from build123d import *

# Parameters (mm, degrees)
SALIENTE_EXTRUIR1_DEPTH = 3
CROQUIS2_R              = 2.5
CROQUIS2_R_2            = 1.1
CORTAR_EXTRUIR1_DEPTH   = 10
REDONDEO1_R             = 5


with BuildPart() as part:
    # Croquis1 → Saliente-Extruir1 (new body)
    with BuildSketch(Plane(origin=(0, 0, 0), x_dir=(1, 0, 0), z_dir=(0, 1, 0))):
        Polygon((-6, 5), (-6, 2.5), (-9, 2.5), (-9, -2.5), (-6, -2.5), (-6, -5), (6, -5), (6, 5), align=None)
    extrude(amount=SALIENTE_EXTRUIR1_DEPTH)

    # Croquis2 → Cortar-Extruir1 (cut)
    with BuildSketch(Plane(origin=(0, 3, 0), x_dir=(1, 0, 0), z_dir=(0, 1, 0))):
        with Locations(Location((1.4, 0, 0), (0, 0, 270))):
            Circle(CROQUIS2_R)
        with Locations(Location((-3.6, 0, 0), (0, 0, 270))):
            Circle(CROQUIS2_R_2)
    extrude(amount=-CORTAR_EXTRUIR1_DEPTH, mode=Mode.SUBTRACT)

    # Redondeo1
    redondeo1_edges = [part.edges().sort_by_distance(p)[0] for p in [
        (6, 1.5, -5),
        (6, 1.5, 5),
    ]]
    fillet(redondeo1_edges, radius=REDONDEO1_R - 0.0001)  # a hair under: the kernel refuses the full size


solid = part.part
Source: CAD feature listing. Evaluate the final solid. Frame: model axes, mm. A direction names the side the tool comes from. Round coordinates to 2 decimals unless told otherwise and drop trailing zeros. Loops run counter-clockwise (first coordinate to the right, second up) from the corner with the lowest first, then second, coordinate; pieces in that order, holes last. Notation, with made-up numbers: (85.5, 83) - (109.5, 83) arc R27 cw to (109.5, 111) - close; hole circle Ø11 at (-15.5, 84.5). An arc over 180 degrees is marked (long way). Write item = value, one per line. Start each with the question number.
Item 1: Reachability of faces 4 (the face through (-8, 1, 2.5)), 5 (the face through (-2.51, 1.52, -0.14)), 6 (the face through (-7, 1, -2.5)) from +Z, -Z, +X, -X, +Y, -Y: full face, straight path, thin tool, end or side. Return the list, or none.
Item 2: Section query B-B on y = 2.35. Count the separate pieces of the cut face and the enclosed holes in it, plus the area to 3 significant figures.
Item 3: Material intervals for line 1 (X direction, y = 2.45, z = 0); line 2 (X direction, y = 2.45, z = -0.75); line 3 (X direction, y = 2.6, z = -1.5), sorted ascending.
Item 4: Section query D-D on x = 0. Output: boundary loops of the cut face in (y, z).
Item 5: First-contact query: pin 1 Ø1.2 at (y, z) = (1, 3.5) entering from -X; pin 2 Ø1.5 at (x, y) = (-7.5, 1) entering from +Z; pin 3 Ø1.5 at (x, y) = (-7, 1) entering from -Z. Flat tips, straight axial feed; report the tip coordinate or a pass-through.
Item 6: Mould query, pull axis X, two halves, no side actions, for faces 1 (the face through (-9, 1, 0)), 2 (the face through (4, 2, -4)), 3 (the face through (-1.04, 1.52, -0.54)). Classes: released by +X, released by -X, zero draft, split by the parting line, or undercut.
Item 7: Section query A-A on x = -3.6. Output: boundary loops of the cut face in (y, z).
Item 8: Section query C-C on z = -0.25. Output: boundary loops of the cut face in (x, y), plus the area to 3 significant figures.
Results list:
q1.face_4 = +Z, -X, +Y, -Y
q1.face_5 = +Y, -Y
q1.face_6 = -Z, -X, +Y, -Y
q2.separate_pieces = 1
q2.enclosed_holes = 2
q2.area = 101 mm²
q3.line_1 = -9 to -4.7, -2.5 to -1.1, 3.9 to 6
q3.line_2 = -9 to -4.4, -2.8 to -0.98, 3.78 to 5.94
q3.line_3 = -9 to -0.6, 3.4 to 5.77
q4.outline = (0, -5) - (3, -5) - (3, -2.07) - (0, -2.07) - close; (0, 2.07) - (3, 2.07) - (3, 5) - (0, 5) - close
q5.pin_1 = -6
q5.pin_2 = 2.5
q5.pin_3 = -2.5
q6.face_1 = released by -X
q6.face_2 = released by +X
q6.face_3 = undercut
q7.outline = (0, -5) - (3, -5) - (3, -1.1) - (0, -1.1) - close; (0, 1.1) - (3, 1.1) - (3, 5) - (0, 5) - close
q8.outline = (-9, 0) - (-4.67, 0) - (-4.67, 3) - (-9, 3) - close; (-2.53, 0) - (-1.09, 0) - (-1.09, 3) - (-2.53, 3) - close; (3.89, 0) - (5.99, 0) - (5.99, 3) - (3.89, 3) - close
q8.area = 23.6 mm²
